```python
from build123d import *

# Parameters (mm, degrees)
F0_W     = 50.8
F0_H     = 50.8
F1_DEPTH = 50.8
F2_R     = 13.0683
F3_DEPTH = 50.8
F4_R     = 16.558312
F5_DEPTH = 12.7
F6_W     = 32.271338
F6_H     = 34.753747
F7_DEPTH = 12.7


with BuildPart() as f1:
    # F0 (on Front) → F1 (new body)
    with BuildSketch(Plane.XZ):
        with Locations((-25.4, 25.4)):
            Rectangle(F0_W, F0_H)
    extrude(amount=F1_DEPTH)

    # F2 (on face) → F3 (cut)
    with BuildSketch(Plane.XY.offset(50.8)):
        with Locations((-26.351742, -25.587924)):
            Circle(F2_R)
    extrude(amount=-F3_DEPTH, mode=Mode.SUBTRACT)

    # F4 (on face) → F5 (join)
    with BuildSketch(Plane.YZ):
        with Locations((-26.086254, 26.009806)):
            Circle(F4_R)
    extrude(amount=F5_DEPTH)

    # F6 (on face) → F7 (join)
    with BuildSketch(Plane.XZ.offset(50.8)):
        with Locations((-25.110537, 25.587923)):
            Rectangle(F6_W, F6_H)
    extrude(amount=F7_DEPTH)


solid = f1.part
```
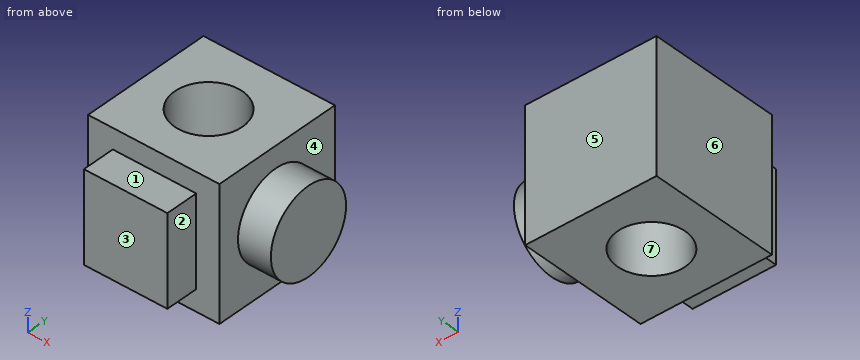
Could you check a few things on this model? Use its own coordinates, in mm. Face numbers are marked on the shaded views. A direction names the side the tool comes from. Coordinates: 2 decimals unless noted, no trailing zeros. Write each loop counter-clockwise with the first axis right and the second up, starting at its lowest first coordinate (ties: lowest second). Pieces come first, ordered by that corner, then holes. Notation, with made-up numbers: (23.5, 8.25) -> (31.5, 8.25) arc R36 cw to (31.5, 45.25) -> close; hole circle Ø5 at (5, 70). An arc over 180 degrees is marked (long way). Return JSON: item names as keys, results as strings.
(1) Imagine slicing it at C-C, the plane z = 19. Please give me the cut outline in (x, y), then the cut area to 4 significant figures.
Numbers:
{"outline": "(-50.8, -50.8) -> (-41.25, -50.8) -> (-41.25, -63.5) -> (-8.97, -63.5) -> (-8.97, -50.8) -> (0, -50.8) -> (0, -41.09) -> (12.7, -41.09) -> (12.7, -11.08) -> (0, -11.08) -> (0, 0) -> (-50.8, 0) -> close; hole circle Ø26.14 at (-26.35, -25.59)", "area": "2,835 mm2"}
(2) I'm going to push flat-ended pins straight in: pin 1 (10 mm diameter, centred on y = -59, z = 25, fed in from +X); pin 2 (2 mm diameter, centred on y = -8, z = 43, fed in from +X); pin 3 (4 mm diameter, centred on x = -4.5, z = 19.5, fed in from -Y). Where does each tip first touch, or does it pass through?
Numbers:
{"pin 1": "stops at x = -8.97", "pin 2": "stops at x = 0", "pin 3": "stops at y = -50.8"}
(3) Which directions (+Z, -Z, +X, -X, +Y, -Y) give clear straight access to the entire face, cutting with the end or side of a thin tool? Please do the marked faces 1, 2, 3 and 4.
Numbers:
{"face 1": "+Z, +X, -X, -Y", "face 2": "+Z, -Z, +X, -Y", "face 3": "+Z, -Z, +X, -X, -Y", "face 4": "+X"}
(4) Imagine slicing it at B-B, the plane y = -18. Please give me the cut outline in (x, z).
Numbers:
{"outline": "(-50.8, 0) -> (-36.99, 0) -> (-36.99, 50.8) -> (-50.8, 50.8) -> close; (-15.71, 0) -> (0, 0) -> (0, 11.56) -> (12.7, 11.56) -> (12.7, 40.46) -> (0, 40.46) -> (0, 50.8) -> (-15.71, 50.8) -> close"}
(5) Imagine slicing it at D-D, the plane x = -11. Please give me the cut outline in (y, z).
Numbers:
{"outline": "(-63.5, 8.21) -> (-50.8, 8.21) -> (-50.8, 0) -> (0, 0) -> (0, 50.8) -> (-50.8, 50.8) -> (-50.8, 42.96) -> (-63.5, 42.96) -> close"}
(6) Imagine slicing it at A-A, the plane x = -34.5. Please give me the cut outline in (y, z), then the cut area to 3 significant figures.
Numbers:
{"outline": "(-63.5, 8.21) -> (-50.8, 8.21) -> (-50.8, 0) -> (-35.8, 0) -> (-35.8, 50.8) -> (-50.8, 50.8) -> (-50.8, 42.96) -> (-63.5, 42.96) -> close; (-15.37, 0) -> (0, 0) -> (0, 50.8) -> (-15.37, 50.8) -> close", "area": "1,980 mm2"}
(7) We'd pull the mould along Y, two halves only. Please class the marked faces 5, 6 and 7: +Y half, -Y half, draft (parallel to the pull), parting line (faces both ways), or undercut.
Numbers:
{"face 5": "+Y half", "face 6": "draft", "face 7": "undercut"}
(8) I need wall thicknesses on L1, parallel to Y at x = -26, z = 3.5; L2, parallel to Z at x = -26, y = -53; L3, parallel to X at y = -6, z = 19. Which ranges of each line are inside material? Lowest first, please.
Numbers:
{"L1": "y = -50.8 to -38.65, -12.52 to 0", "L2": "z = 8.21 to 42.96", "L3": "x = -50.8 to 0"}
